Check sheet for the modelled part. Datum: model origin and axes. Units: mm. Face numbers are marked on the shaded views. A direction names the side the tool comes from. Give positions to 0.01 mm unless a question says otherwise; leave off trailing zeros. Write each loop counter-clockwise with the first axis right and the second up, starting at its lowest first coordinate (ties: lowest second). Pieces come first, ordered by that corner, then holes. Notation, with made-up numbers: (70.25, 45) -> (96.25, 45) arc R21 ccw to (96.25, 76) -> close; hole circle Ø3 at (-21, 20.25). An arc over 180 degrees is marked (long way). Return JSON: item names as keys, results as strings.
from build123d import *

# Parameters (mm, degrees)
F0_R      = 4.7752
F0_R_2    = 6.3627
F1_DEPTH  = 8.509
F2_DEPTH  = 80.4418
F3_R      = 4.7752
F4_DEPTH  = 30.5308
F5_R      = 4.7752
F5_R_2    = 6.3627
F6_DEPTH  = 8.509
F7_R      = 6.3627
F8_DEPTH  = 24.5364
F9_R      = 2.38125
F10_DEPTH = 10.414


with BuildPart() as f1:
    # F0 (on Right) → F1 (new body)
    with BuildSketch(Plane.YZ):
        with BuildLine():
            ThreePointArc((-7.700766, -25.608431), (-5.713574, -29.396277), (-1.774759, -31.064344))
            ThreePointArc((-1.774759, -31.064344), (1.50712, -31.078478), (4.772233, -30.746854))
            ThreePointArc((4.772233, -30.746854), (6.475424, -29.874653), (7.323086, -28.159117))
            Line((7.323086, -28.159117), (9.301448, -14.082338))
            ThreePointArc((9.301448, -14.082338), (11.768125, -9.894752), (16.473399, -8.677885))
            Line((16.473399, -8.677885), (23.647041, -9.686075))
            ThreePointArc((23.647041, -9.686075), (28.357354, -8.465408), (30.820737, -4.269122))
            ThreePointArc((30.820737, -4.269122), (0, 31.115), (-30.820737, -4.269122))
            ThreePointArc((-30.820737, -4.269122), (-28.357354, -8.465408), (-23.647041, -9.686075))
            Line((-23.647041, -9.686075), (-16.492232, -8.680532))
            ThreePointArc((-16.492232, -8.680532), (-11.786957, -9.897399), (-9.32028, -14.084985))
            Line((-9.32028, -14.084985), (-7.700766, -25.608431))
        make_face()
        with Locations((0, -23.8252)):
            Circle(F0_R, mode=Mode.SUBTRACT)
        Circle(F0_R_2, mode=Mode.SUBTRACT)
        Circle(F0_R_2)
    extrude(amount=F1_DEPTH)

    # F0 (on Right) → F2 (join)
    with BuildSketch(Plane.YZ):
        Circle(F0_R_2)
    extrude(amount=-F2_DEPTH)

    # F3 (on face) → F4 (join)
    with BuildSketch(Plane(origin=(0, 0, 0), x_dir=(0, -1, 0), z_dir=(-1, 0, 0))):
        with Locations((0, -23.8252)):
            Circle(F3_R)
    extrude(amount=-F4_DEPTH)

    # F5 (on face) → F6 (join)
    with BuildSketch(Plane.YZ.offset(30.5308)):
        with BuildLine():
            ThreePointArc((26.729671, -10.11931), (28.843815, -9.637583), (30.102707, -7.87212))
            ThreePointArc((30.102707, -7.87212), (0, 31.115), (-30.102707, -7.87212))
            ThreePointArc((-30.102707, -7.87212), (-28.843815, -9.637583), (-26.729671, -10.11931))
            Line((-26.729671, -10.11931), (-16.492232, -8.680532))
            ThreePointArc((-16.492232, -8.680532), (-11.786957, -9.897399), (-9.32028, -14.084985))
            Line((-9.32028, -14.084985), (-7.797371, -24.921049))
            Line((-7.797371, -24.921049), (-7.342719, -28.156062))
            ThreePointArc((-7.342719, -28.156062), (-6.495815, -29.87083), (-4.793998, -30.743468))
            ThreePointArc((-4.793998, -30.743468), (0, -31.115), (4.793998, -30.743468))
            ThreePointArc((4.793998, -30.743468), (6.495815, -29.87083), (7.342719, -28.156062))
            Line((7.342719, -28.156062), (7.797371, -24.921049))
            Line((7.797371, -24.921049), (9.32028, -14.084985))
            ThreePointArc((9.32028, -14.084985), (11.786957, -9.897399), (16.492232, -8.680532))
            Line((16.492232, -8.680532), (26.729671, -10.11931))
        make_face()
        with Locations((0, -23.8252)):
            Circle(F5_R, mode=Mode.SUBTRACT)
        Circle(F5_R_2, mode=Mode.SUBTRACT)
    extrude(amount=-F6_DEPTH)

    # F7 (on face) → F8 (join)
    with BuildSketch(Plane(origin=(22.0218, 0, 0), x_dir=(0, -1, 0), z_dir=(-1, 0, 0))):
        Circle(F7_R)
    extrude(amount=-F8_DEPTH)

    # F9 (on face) → F10 (join)
    with BuildSketch(Plane.YZ.offset(46.5582)):
        Circle(F9_R)
    extrude(amount=F10_DEPTH)


solid = f1.part
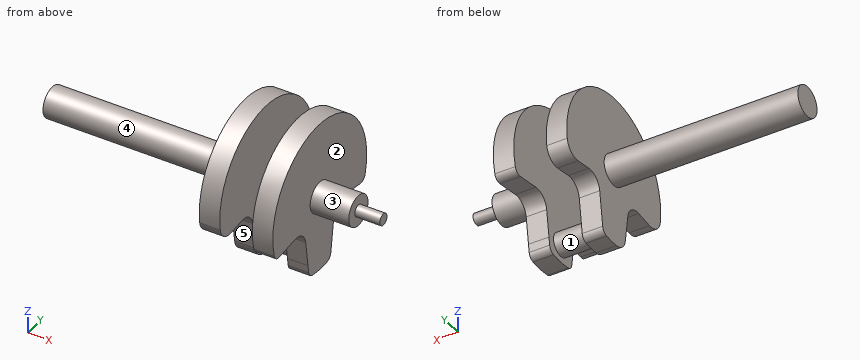
(1) Thickness scan on L1, parallel to X at y = 16.5, z = 0; L2, parallel to Z at x = 46, y = 3.5; L3, parallel to Z at x = -9.5, y = 4.5. Record the ranges inside material, lowest first.
Reply:
{"L1": "0 to 8.51, 22.02 to 30.53", "L2": "-5.31 to 5.31", "L3": "-4.5 to 4.5"}
(2) Set-up check for the marked faces 4 and 5: record each of +Z, -Z, +X, -X, +Y, -Y from which the full face is reachable in a straight line by a thin tool's end or side.
Reply:
{"face 4": "-X", "face 5": "-Z, +X, -X, -Y"}
(3) Cross-section at B-B on y = -15. Enter the section's corners in (x, z), then the cut area to 3 significant figures.
Reply:
{"outline": "(0, -8.65) -> (8.51, -8.65) -> (8.51, 27.26) -> (0, 27.26) -> close; (22.02, -8.65) -> (30.53, -8.65) -> (30.53, 27.26) -> (22.02, 27.26) -> close", "area": "611 mm^2"}
(4) Cross-section at C-C on y = 0. Enter the section's corners in (x, z) (3 decimals).
Reply:
{"outline": "(-80.442, -6.363) -> (0, -6.363) -> (0, -31.115) -> (8.509, -31.115) -> (8.509, -28.6) -> (22.022, -28.6) -> (22.022, -31.115) -> (30.531, -31.115) -> (30.531, -6.363) -> (46.558, -6.363) -> (46.558, -2.381) -> (56.972, -2.381) -> (56.972, 2.381) -> (46.558, 2.381) -> (46.558, 6.363) -> (30.531, 6.363) -> (30.531, 31.115) -> (22.022, 31.115) -> (22.022, -19.05) -> (8.509, -19.05) -> (8.509, 31.115) -> (0, 31.115) -> (0, 6.363) -> (-80.442, 6.363) -> close"}
(5) Release check for a two-part mould opening along X. For the marked faces 1, 2 and 3 record: pulls with the +X half, pulls with the -X half, needs draft (parallel to the pull), parting line crosses it, or undercut.
Reply:
{"face 1": "undercut", "face 2": "pulls with the +X half", "face 3": "needs draft"}
(6) Depth check by flat-ended pin: pin 1 Ø5 at (x, z) = (-48.5, -4.5) entering from +Y; pin 2 Ø2 at (x, y) = (7, 22) entering from +Z; pin 3 Ø1 at (y, z) = (-12.5, -2) entering from -X. Enter the tip coordinate at first touch or a pass-through.
Reply:
{"pin 1": "y = 6.04", "pin 2": "z = 22.96", "pin 3": "x = 0"}
(7) Cross-section at D-D on z = 21. Enter the section's corners in (x, y), then the cut area to 3 significant figures.
Reply:
{"outline": "(0, -22.96) -> (8.51, -22.96) -> (8.51, 22.96) -> (0, 22.96) -> close; (22.02, -22.96) -> (30.53, -22.96) -> (30.53, 22.96) -> (22.02, 22.96) -> close", "area": "781 mm^2"}
(8) Cross-section at A-A on z = 0. Enter the section's corners in (x, y) (3 decimals), then the cut area to 3 significant figures.
Reply:
{"outline": "(-80.442, -6.363) -> (0, -6.363) -> (0, -31.115) -> (8.509, -31.115) -> (8.509, 31.115) -> (0, 31.115) -> (0, 6.363) -> (-80.442, 6.363) -> close; (22.022, -31.115) -> (30.531, -31.115) -> (30.531, -6.363) -> (46.558, -6.363) -> (46.558, -2.381) -> (56.972, -2.381) -> (56.972, 2.381) -> (46.558, 2.381) -> (46.558, 6.363) -> (30.531, 6.363) -> (30.531, 31.115) -> (22.022, 31.115) -> close", "area": "2,340 mm^2"}
